```python
from build123d import *

# Parameters (mm, degrees)
F0_W     = 15
F0_H     = 33
F0_R     = 1.715
F1_DEPTH = 3
F2_W     = 15
F2_H     = 20
F2_R     = 2.25
F3_DEPTH = 3
F4_W     = 15
F4_H     = 18.209726
F4_R     = 1.5
F5_DEPTH = 3


with BuildPart() as f1:
    # F0 (on Top) → F1 (new body)
    with BuildSketch(Plane.XY):
        Rectangle(F0_W, F0_H)
        with Locations((-2.285, -4.955)):
            Circle(F0_R, mode=Mode.SUBTRACT)
        with Locations((-2.285, 12.485)):
            Circle(F0_R, mode=Mode.SUBTRACT)
    extrude(amount=F1_DEPTH)

    # F2 (on face) → F3 (join)
    with BuildSketch(Plane(origin=(0, 16.5, 0), x_dir=(-1, 0, 0), z_dir=(0, 1, 0))):
        with Locations((0, -7)):
            Rectangle(F2_W, F2_H)
        with Locations((-3.308824, -12.25)):
            Circle(F2_R, mode=Mode.SUBTRACT)
        with Locations((3.308824, -4.75)):
            Circle(F2_R, mode=Mode.SUBTRACT)
    extrude(amount=F3_DEPTH)

    # F4 (on face) → F5 (join)
    with BuildSketch(Plane.XZ.offset(16.5)):
        with Locations((0, 12.104863)):
            Rectangle(F4_W, F4_H)
        with Locations((0, 11.881463)):
            Circle(F4_R, mode=Mode.SUBTRACT)
    extrude(amount=-F5_DEPTH)


solid = f1.part
```
Check sheet for the modelled part. Datum: model origin and axes. Units: mm. A direction names the side the tool comes from. Round coordinates to 2 decimals unless told otherwise and drop trailing zeros. Loops run counter-clockwise (first coordinate to the right, second up) from the corner with the lowest first, then second, coordinate; pieces in that order, holes last. Notation, with made-up numbers: (-5.5, 81.25) - (37.5, 81.25) arc R16 cw to (37.5, 99.25) - close; hole circle Ø6 at (15, -17.75). An arc over 180 degrees is marked (long way). Answer as a JSON object with one key per item and string values. Group by question number.
Q1. Scan lines: line 1 along Z through (x, y) = (0, -15.5); line 2 along Z through (x, y) = (-2, 2); line 3 along Z through (x, y) = (-2.5, -15). Record each from-to range of solid material in increasing order. Write a range as [from, to].
Q2. Sectioned sample at A-A, the plane x = 0. Enter the section's corners in (y, z).
Q3. Sectioned sample at C-C, the plane x = -6.25. Enter the section's corners in (y, z).
Q4. Sectioned sample at B-B, the plane z = -4.75. Enter the section's corners in (x, y), plus the area to 3 significant figures.
Q5. Gauge pin test, flat ends, axial feed: P1, Ø4, axis at x = 3.31, z = -12.25, coming from the +Y side; P2, Ø4, axis at x = -2.285, y = -4.955, coming from the +Z side; P3, Ø3.5, axis at x = 0, z = 11.88, coming from the +Y side; P4, Ø6, axis at x = -1, y = 1, coming from the -Z side. Record the tip position at first contact, or that the pin passes through.
Q6. Sectioned sample at D-D, the plane y = 6. Enter the section's corners in (x, z).
Q7. Set-up check for faces 1 (the face through (-2, -13.5, 12)), 2 (the face through (-2.66, -6.63, 1.48)), 3 (the face through (0, 16.5, -8)): record each of +Z, -Z, +X, -X, +Y, -Y from which the full face is reachable in a straight line by a thin tool's end or side.
Q8. Mould release check, pull along X, two halves, no side actions. Record for faces 4 (the face through (-1.06, 17.98, -4.65)), 5 (the face through (1, -15, 13)), 6 (the face through (7.5, 1, 2)), 7 (the face through (0, 3, 3)): released by +X, released by -X, zero draft, split by the parting line, or undercut.
Solution:
{
 "1": {"line 1": "z = [0, 10.38], [13.38, 21.21]", "line 2": "z = [0, 3]", "line 3": "z = [0, 21.21]"},
 "2": {"outline": "(-16.5, 0) - (16.5, 0) - (16.5, -17) - (19.5, -17) - (19.5, 3) - (-13.5, 3) - (-13.5, 10.38) - (-16.5, 10.38) - close; (-16.5, 13.38) - (-13.5, 13.38) - (-13.5, 21.21) - (-16.5, 21.21) - close"},
 "3": {"outline": "(-16.5, 0) - (16.5, 0) - (16.5, -17) - (19.5, -17) - (19.5, 3) - (-13.5, 3) - (-13.5, 21.21) - (-16.5, 21.21) - close"},
 "4": {"outline": "(-7.5, 16.5) - (-5.56, 16.5) - (-5.56, 19.5) - (-7.5, 19.5) - close; (-1.06, 16.5) - (7.5, 16.5) - (7.5, 19.5) - (-1.06, 19.5) - close", "area": "31.5 mm²"},
 "5": {"P1": "passes through", "P2": "stops at z = 3", "P3": "stops at y = -13.5", "P4": "stops at z = 0"},
 "6": {"outline": "(-7.5, 0) - (7.5, 0) - (7.5, 3) - (-7.5, 3) - close"},
 "7": {"face 1": "+Z, +X, -X, +Y", "face 2": "+Z, -Z", "face 3": "-Z, +X, -X, -Y"},
 "8": {"face 4": "undercut", "face 5": "undercut", "face 6": "released by +X", "face 7": "zero draft"}
}
